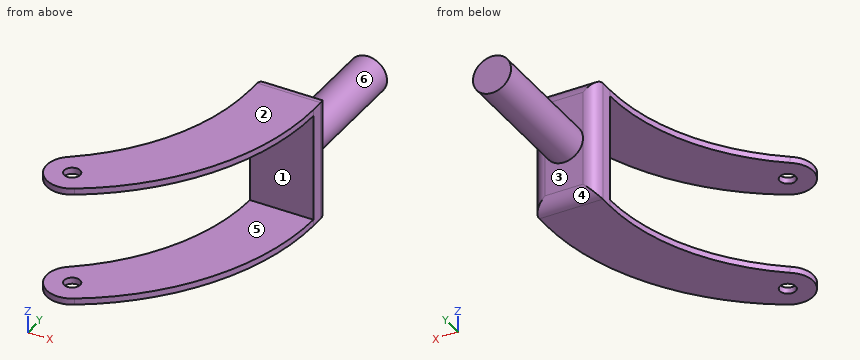
from build123d import *

# Parameters (mm, degrees)
SKETCH_R     = 3.969
PAD_DEPTH    = 30.1625
SKETCH001_W  = 127
SKETCH001_H  = 53.975
POCKET_DEPTH = 79.376
SKETCH002_R  = 9.525
PAD001_DEPTH = 63.5
FILLET_R     = 6.3


with BuildPart() as part:
    # Sketch → Pad (new body, symmetric)
    with BuildSketch(Plane.XY):
        with BuildLine():
            ThreePointArc((-7.075094, 10.546707), (-10.546707, -7.075094), (7.075094, -10.546707))
            ThreePointArc((7.075094, -10.546707), (50.749937, 34.535315), (66.675, 95.25))
            Line((66.675, 95.25), (66.675, 107.95))
            Line((34.925, 107.95), (66.675, 107.95))
            Line((34.925, 95.25), (34.925, 107.95))
            ThreePointArc((-7.075094, 10.546707), (23.848498, 47.977768), (34.925, 95.25))
        make_face()
        Circle(SKETCH_R, mode=Mode.SUBTRACT)
    extrude(amount=PAD_DEPTH, both=True)

    # Sketch001 (on Face4 of Pad) → Pocket (cut, through all)
    with BuildSketch(Plane.YZ.offset(66.675)):
        with Locations((31.75, 0)):
            Rectangle(SKETCH001_W, SKETCH001_H)
    extrude(amount=-POCKET_DEPTH, mode=Mode.SUBTRACT)

    # Sketch002 (on Face8 of Pocket) → Pad001 (join)
    with BuildSketch(Plane(origin=(0, 107.95, 0), x_dir=(-1, 0, 0), z_dir=(0, 1, 0))):
        with Locations((-50.8, 0)):
            Circle(SKETCH002_R)
    extrude(amount=PAD001_DEPTH)

    # Fillet
    fillet_edges = [part.edges().sort_by_distance(p)[0] for p in [
        (50.8, 107.95, 30.1625),
        (66.675, 107.95, 0),
        (34.925, 107.95, 0),
        (50.8, 107.95, -30.1625),
    ]]
    fillet(fillet_edges, radius=FILLET_R)


solid = part.part
Could you check a few things on this model? Use its own coordinates, in mm. Face numbers are marked on the shaded views. A direction names the side the tool comes from. Coordinates: 2 decimals unless noted, no trailing zeros. Order: outer loops, then holes, each group sorted by start corner. A loop starts at its lowest first (then second) coordinate and runs counter-clockwise, first axis right, second up. Notation, with made-up numbers: (-6.5, 89) -> (1.5, 89) arc R22 cw to (1.5, 97) -> close; hole circle Ø4 at (76.5, -19.75). An arc over 180 degrees is marked (long way). One line per question, with ' | ' between items.
Q1. If I drill on L1, parallel to Z at x = 12, y = 24; L2, parallel to Y at x = 59, z = -9; L3, parallel to Y at x = 0, z = -27.7, over which ranges is the centre line in solid material (lowest first)?
Return value:
L1: -30.16 to -26.99, 26.99 to 30.16 | L2: 95.25 to 107.95 | L3: -12.7 to -3.97, 3.97 to 16.43
Q2. Imagine slicing it at B-B on y = 0. Please give me the cut outline in (x, z), and give its area (3 significant figures).
Return value:
outline: (-12.7, -30.16) -> (-3.97, -30.16) -> (-3.97, -26.99) -> (-12.7, -26.99) -> close; (-12.7, 26.99) -> (-3.97, 26.99) -> (-3.97, 30.16) -> (-12.7, 30.16) -> close; (3.97, -30.16) -> (21.9, -30.16) -> (21.9, -26.99) -> (3.97, -26.99) -> close; (3.97, 26.99) -> (21.9, 26.99) -> (21.9, 30.16) -> (3.97, 30.16) -> close | area: 169 mm²
Q3. I'm going to push flat-ended pins straight in: P1, Ø16, axis at x = 51.5, z = -6, coming from the -Y side; P2, Ø7, axis at y = 99, z = -3, coming from the -X side (3 decimals); P3, Ø2, axis at y = 144.5, z = -6.5, coming from the +X side. Where does each tip first touch, or does it pass through?
Return value:
P1: y = 95.25 | P2: x = 34.925 | P3: x = 58.58
Q4. On a 3-axis mill with a long thin cutter (end or side, diameter ignored), from which of +Z, -Z, +X, -X, +Y, -Y can I reach the whole of each face in a straight line? I mean the marked faces 1 and 2. Say none if no direction works.
Return value:
face 1: +X, -X, -Y | face 2: +Z, +X, -X, +Y, -Y
Q5. Imagine slicing it at C-C on y = 86. Please give me the cut outline in (x, z).
Return value:
outline: (34.52, -30.16) -> (66.33, -30.16) -> (66.33, -26.99) -> (34.52, -26.99) -> close; (34.52, 26.99) -> (66.33, 26.99) -> (66.33, 30.16) -> (34.52, 30.16) -> close
Q6. Imagine slicing it at A-A on x = 0. Please give me the cut outline in (y, z), and give its area (3 significant figures).
Return value:
outline: (-12.7, -30.16) -> (-3.97, -30.16) -> (-3.97, -26.99) -> (-12.7, -26.99) -> close; (-12.7, 26.99) -> (-3.97, 26.99) -> (-3.97, 30.16) -> (-12.7, 30.16) -> close; (3.97, -30.16) -> (16.43, -30.16) -> (16.43, -26.99) -> (3.97, -26.99) -> close; (3.97, 26.99) -> (16.43, 26.99) -> (16.43, 30.16) -> (3.97, 30.16) -> close | area: 135 mm²
Q7. Thinking about a two-plate mould opening in Z: for the marked faces 3, 4, 5 and 6, which applies, pulls with the +Z half, pulls with the -Z half, needs draft (parallel to the pull), parting line crosses it, or undercut?
Return value:
face 3: needs draft | face 4: pulls with the -Z half | face 5: undercut | face 6: parting line crosses it
Q8. Imagine slicing it at D-D on z = 0. Please give me the cut outline in (x, y) (3 decimals).
Return value:
outline: (34.925, 95.25) -> (66.675, 95.25) -> (66.675, 101.65) arc R6.3 ccw to (60.375, 107.95) -> (60.325, 107.95) -> (60.325, 171.45) -> (41.275, 171.45) -> (41.275, 107.95) -> (41.225, 107.95) arc R6.3 ccw to (34.925, 101.65) -> close
